from build123d import *

# Parameters (mm, degrees)
SKETCH1_W                     = 190.5
SKETCH1_H                     = 101.6
BOSS_EXTRUDE1_DEPTH           = 1.5875
CONVERT_SOLID1_START          = -95.25
CONVERT_SOLID1_OUTLINE_W      = 3.175
CONVERT_SOLID1_OUTLINE_H      = 101.6
CONVERT_SOLID1_DEPTH          = 190.5
CUT_EXTRUDE5_START            = -4.7625
CUT_EXTRUDE5_DEPTH            = 4.7625
FILLET3_R                     = 25.4
FILLET4_R                     = 25.4
FILLET5_R                     = 25.4
FILLET6_R                     = 25.4
SKETCH30_R                    = 12.770921212
CUT_EXTRUDE6_DEPTH            = 38.1
SKETCH35_W                    = 139.601875342
SKETCH35_H                    = 6.35
CUT_EXTRUDE7_DEPTH            = 0.254
EDGE_FLANGE1_STRIP_W          = 39.05
EDGE_FLANGE1_STRIP_H          = 4.7625
EDGE_FLANGE1_STRIP_CUT_DEPTH  = 25.449062329
EDGE_FLANGE1_RELIEF_W         = 41.43125
EDGE_FLANGE1_RELIEF_H         = 2.38125
EDGE_FLANGE1_RELIEF_CUT_DEPTH = 4.7625
EDGE_FLANGE1_DEPTH            = 25.449062329
EDGE_FLANGE2_STRIP_W          = 39.05
EDGE_FLANGE2_STRIP_H          = 4.7625
EDGE_FLANGE2_STRIP_CUT_DEPTH  = 25.449062329
EDGE_FLANGE2_RELIEF_W         = 41.43125
EDGE_FLANGE2_RELIEF_H         = 2.38125
EDGE_FLANGE2_RELIEF_CUT_DEPTH = 4.7625
EDGE_FLANGE2_DEPTH            = 25.449062329


# Read off the part's stored shape, not the designer's step: Convert-Solid1, Cut-Extrude5
# Sheet-metal steps are written as plain solids
with BuildPart() as part:
    # Sketch1 → Boss-Extrude1 (new body)
    with BuildSketch(Plane(origin=(0, 0, 0), x_dir=(1, 0, 0), z_dir=(0, 1, 0))):
        Rectangle(SKETCH1_W, SKETCH1_H)
    extrude(amount=BOSS_EXTRUDE1_DEPTH)

    # Convert-Solid1 outline → Convert-Solid1 (add)
    with BuildSketch(Plane.YZ.offset(CONVERT_SOLID1_START)):
        with Locations((-1.5875, 0)):
            Rectangle(CONVERT_SOLID1_OUTLINE_W, CONVERT_SOLID1_OUTLINE_H)
    extrude(amount=CONVERT_SOLID1_DEPTH)

    # Cut-Extrude5 outline → Cut-Extrude5 (cut)
    with BuildSketch(Plane(origin=(0, 1.5875, 0), x_dir=(1, 0, 0), z_dir=(0, 1, 0)).offset(CUT_EXTRUDE5_START)):
        with BuildLine():
            Line((95.25, -50.8), (95.25, 0))
            add(Edge.make_bspline(
                [(95.25, 0), (74.104329576, -30.281671419), (43.45324244, -50.8)],
                knots=[0, 0, 0, 1, 1, 1], degree=2))
            Line((43.45324244, -50.8), (95.25, -50.8))
        make_face()
        with BuildLine():
            Line((-95.25, -50.8), (-43.45324244, -50.8))
            add(Edge.make_bspline(
                [(-43.45324244, -50.8), (-74.104329576, -30.281671419), (-95.25, 0)],
                knots=[0, 0, 0, 1, 1, 1], degree=2))
            Line((-95.25, 0), (-95.25, -50.8))
        make_face()
    extrude(amount=CUT_EXTRUDE5_DEPTH, mode=Mode.SUBTRACT)

    # Fillet3
    fillet3_edges = [part.edges().sort_by_distance(p)[0] for p in [
        (-95.25, -0.79375, 0),
    ]]
    fillet(fillet3_edges, radius=FILLET3_R)

    # Fillet4
    fillet4_edges = [part.edges().sort_by_distance(p)[0] for p in [
        (-43.45324244, -0.79375, 50.8),
    ]]
    fillet(fillet4_edges, radius=FILLET4_R)

    # Fillet5
    fillet5_edges = [part.edges().sort_by_distance(p)[0] for p in [
        (43.45324244, -0.79375, 50.8),
    ]]
    fillet(fillet5_edges, radius=FILLET5_R)

    # Fillet6
    fillet6_edges = [part.edges().sort_by_distance(p)[0] for p in [
        (95.25, -0.79375, 0),
    ]]
    fillet(fillet6_edges, radius=FILLET6_R)

    # Sketch30 → Cut-Extrude6 (cut)
    with BuildSketch(Plane(origin=(0, -3.175, 0), x_dir=(-1, 0, 0), z_dir=(0, -1, 0))):
        with Locations(Location((0, -25.504506424, 0), (0, 0, 90))):
            Circle(SKETCH30_R)
    extrude(amount=-CUT_EXTRUDE6_DEPTH, mode=Mode.SUBTRACT)

    # Sketch35 → Cut-Extrude7 (cut)
    with BuildSketch(Plane(origin=(0, 0, -50.8), x_dir=(-1, 0, 0), z_dir=(0, 0, -1))):
        Rectangle(SKETCH35_W, SKETCH35_H)
    extrude(amount=-CUT_EXTRUDE7_DEPTH, mode=Mode.SUBTRACT)

    # Edge-Flange1 strip (across the edge) → Edge-Flange1 strip cut (cut)
    with BuildSketch(Plane(origin=(95.25, 1.5875, -50.8), x_dir=(0, 0, 1), z_dir=(-1, 0, 0))):
        with Locations((-4.7625, -2.38125)):
            Rectangle(EDGE_FLANGE1_STRIP_W, EDGE_FLANGE1_STRIP_H)
    extrude(amount=EDGE_FLANGE1_STRIP_CUT_DEPTH, mode=Mode.SUBTRACT)

    # Edge-Flange1 relief (on the sheet) → Edge-Flange1 relief cut (cut)
    with BuildSketch(Plane(origin=(95.25, 1.5875, -36.0375), x_dir=(0, 0, 1), z_dir=(0, 1, 0))):
        with Locations((-18.334375, -26.639687329)):
            Rectangle(EDGE_FLANGE1_RELIEF_W, EDGE_FLANGE1_RELIEF_H)
    extrude(amount=-EDGE_FLANGE1_RELIEF_CUT_DEPTH, mode=Mode.SUBTRACT)

    # Edge-Flange1 section (across the edge) → Edge-Flange1 (add)
    with BuildSketch(Plane(origin=(95.25, 1.5875, -50.8), x_dir=(0, 0, 1), z_dir=(-1, 0, 0))):
        with BuildLine():
            Line((0, 10), (0, 33.3375))
            Line((0, 33.3375), (4.7625, 33.3375))
            Line((4.7625, 33.3375), (4.7625, 10))
            ThreePointArc((4.7625, 10), (7.691432188, 2.928932188), (14.7625, 0))
            Line((14.7625, 0), (14.7625, -4.7625))
            ThreePointArc((14.7625, -4.7625), (4.323836143, -0.438663857), (0, 10))
        make_face()
    extrude(amount=EDGE_FLANGE1_DEPTH)

    # Edge-Flange2 strip (across the edge) → Edge-Flange2 strip cut (cut)
    with BuildSketch(Plane(origin=(-69.800937671, 1.5875, -50.8), x_dir=(0, 0, 1), z_dir=(-1, 0, 0))):
        with Locations((-4.7625, -2.38125)):
            Rectangle(EDGE_FLANGE2_STRIP_W, EDGE_FLANGE2_STRIP_H)
    extrude(amount=EDGE_FLANGE2_STRIP_CUT_DEPTH, mode=Mode.SUBTRACT)

    # Edge-Flange2 relief (on the sheet) → Edge-Flange2 relief cut (cut)
    with BuildSketch(Plane(origin=(-69.800937671, 1.5875, -36.0375), x_dir=(0, 0, 1), z_dir=(0, 1, 0))):
        with Locations((-18.334375, 1.190625)):
            Rectangle(EDGE_FLANGE2_RELIEF_W, EDGE_FLANGE2_RELIEF_H)
    extrude(amount=-EDGE_FLANGE2_RELIEF_CUT_DEPTH, mode=Mode.SUBTRACT)

    # Edge-Flange2 section (across the edge) → Edge-Flange2 (add)
    with BuildSketch(Plane(origin=(-69.800937671, 1.5875, -50.8), x_dir=(0, 0, 1), z_dir=(-1, 0, 0))):
        with BuildLine():
            Line((0, 10), (0, 33.3375))
            Line((0, 33.3375), (4.7625, 33.3375))
            Line((4.7625, 33.3375), (4.7625, 10))
            ThreePointArc((4.7625, 10), (7.691432188, 2.928932188), (14.7625, 0))
            Line((14.7625, 0), (14.7625, -4.7625))
            ThreePointArc((14.7625, -4.7625), (4.323836143, -0.438663857), (0, 10))
        make_face()
    extrude(amount=EDGE_FLANGE2_DEPTH)


solid = part.part
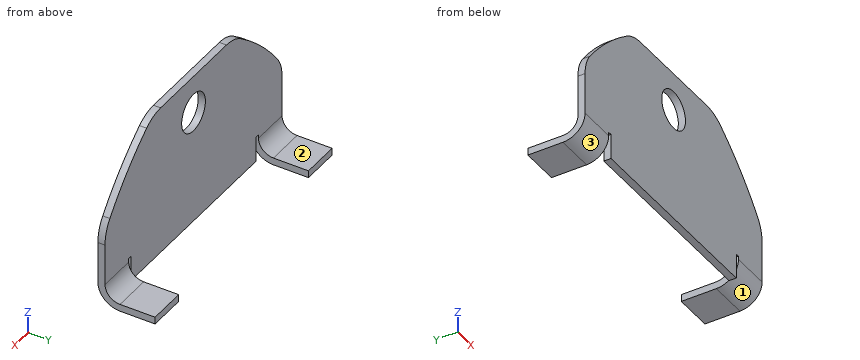
CAD build for the part. Positions are in the model's coordinates, mm. Face numbers are marked on the shaded views. A direction names the side the tool comes from. Give positions to 0.01 mm unless a question says otherwise; leave off trailing zeros. Order: outer loops, then holes, each group sorted by start corner. A loop starts at its lowest first (then second) coordinate and runs counter-clockwise, first axis right, second up. Notation, with made-up numbers: (5, 36) - (48, 36) arc R21 cw to (48, 44) - close; hole circle Ø8 at (11.25, 87.25). An arc over 180 degrees is marked (long way). Answer in a Markdown table with one row per item.
1. Saw through at B-B, the plane x = 0. Give the cut face in (y, z) (1 decimal).
Data:
| item | result |
|---|---|
| outline | (-3.2, -50.5) - (1.6, -50.5) - (1.6, 12.7) - (-3.2, 12.7) - close; (-3.2, 38.3) - (1.6, 38.3) - (1.6, 50.8) - (-3.2, 50.8) - close |
2. Saw through at A-A, the plane y = 20.5. Give the cut face in (x, z).
Data:
| item | result |
|---|---|
| outline | (-95.25, -50.8) - (-69.8, -50.8) - (-69.8, -46.04) - (-95.25, -46.04) - close; (69.8, -50.8) - (95.25, -50.8) - (95.25, -46.04) - (69.8, -46.04) - close |
3. Tool access for the marked faces 1, 2 and 3: list every direction of +Z, -Z, +X, -X, +Y, -Y with a clear straight run to the whole face (end or side of a thin tool).
Data:
| item | result |
|---|---|
| face 1 | -Z, +X, -Y |
| face 2 | +Z, +X, -X, +Y |
| face 3 | -Z, -X, -Y |
4. Flat gauge pins, fed straight in: pin 1 (7 mm diameter, centred on x = -83, y = 23.5, fed in from +Z); pin 2 (5 mm diameter, centred on y = 13.5, z = -42.5, fed in from -X); pin 3 (4 mm diameter, centred on x = -11, y = 0, fed in from -Z); pin 4 (1.2 mm diameter, centred on x = 69, y = -1.5, fed in from -Z). Where does each tip first touch, or does it go through?
Data:
| item | result |
|---|---|
| pin 1 | stops at z = -46.04 |
| pin 2 | passes through |
| pin 3 | stops at z = -50.55 |
| pin 4 | stops at z = -33.66 |
5. Probe probe 1 along Y at (x, z) = (-3, 6.5) (1 decimal); probe 2 along X at (y, z) = (2.5, -40.5); probe 3 along Z at (x, y) = (-76.5, 13.5). List the from-to ranges inside material, lowest first. Write a range as [from, to].
Data:
| item | result |
|---|---|
| probe 1 | y = [-3.2, 1.6] |
| probe 2 | x = [-95.25, -69.8], [69.8, 95.25] |
| probe 3 | z = [-50.8, -46.04] |
